Geometry check sheet. Reference: drawing and pictorial views, mm from the part's lowest x, y, z. Round coordinates to 2 decimals unless told otherwise and drop trailing zeros. Write each loop counter-clockwise with the first axis right and the second up, starting at its lowest first coordinate (ties: lowest second). Pieces come first, ordered by that corner, then holes. Notation, with made-up numbers: (-10.5, 33.5) -> (9.5, 33.5) arc R26 cw to (9.5, 47.5) -> close; hole circle Ø10 at (-8, 13). An arc over 180 degrees is marked (long way). Answer as a JSON object with one key per item and string values. Group by question number.
(1) Sectioned sample at D-D on x = 22. Record the cut outline in (y, z).
(2) Sectioned sample at A-A on x = 15.24. Record the cut outline in (y, z) (3 decimals).
(3) Draft check along X on the marked faces 1, 2, 3 and 4. Enter one of: released by +X, released by -X, zero draft, split by the parting line, or undercut.
(4) Scan lines: L1, parallel to Y at x = 15.24, z = 3.3 (3 decimals); L2, parallel to X at y = 28.5, z = 0.45; L3, parallel to X at y = 29.5, z = 3.4. Record each from-to range of solid material in increasing order. Write a range as from..to.
(5) Sectioned sample at B-B on z = 0.45. Record the cut outline in (x, y) (3 decimals), and give its area (3 significant figures).
(6) Gauge pin test, flat end, axial feed: pin 1 Ø1 at (x, z) = (18, 0.5) entering from -Y. Record the tip position at first contact, or that the pin passes through.
(7) Sectioned sample at C-C on y = 35.5. Record the cut outline in (x, z).
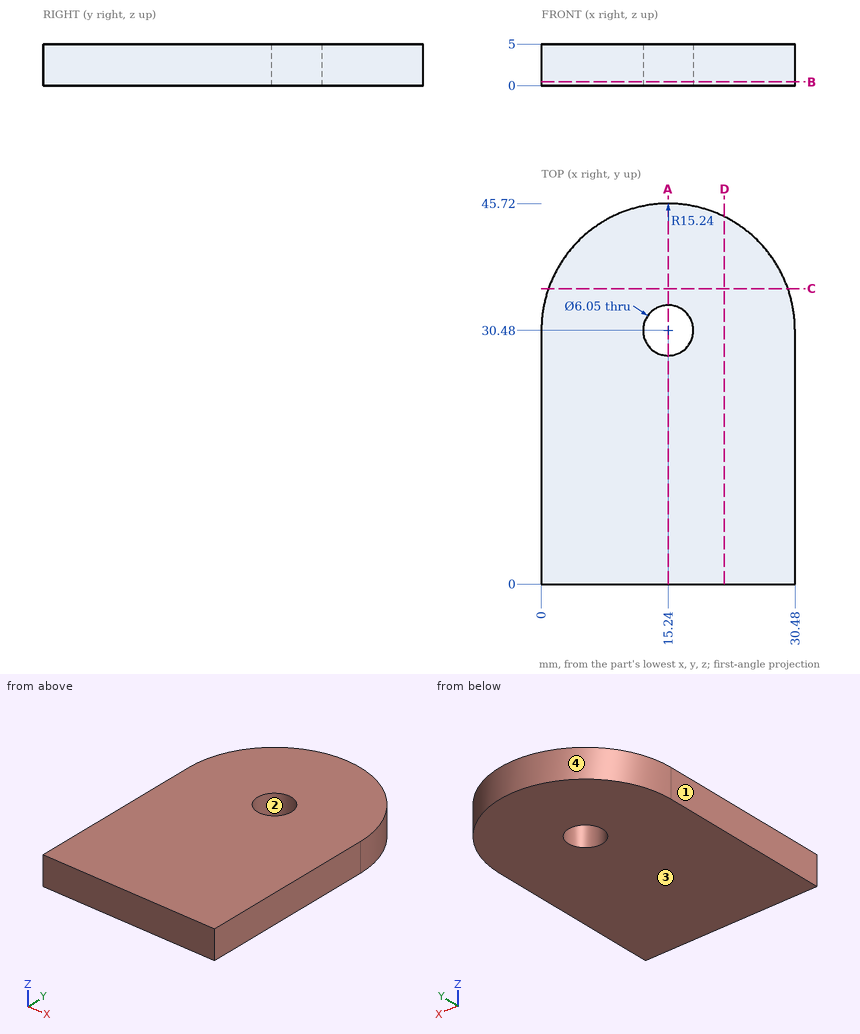
Computed values:
{
 "1": {"outline": "(0, 0) -> (44.14, 0) -> (44.14, 5) -> (0, 5) -> close"},
 "2": {"outline": "(0, 0) -> (27.455, 0) -> (27.455, 5) -> (0, 5) -> close; (33.505, 0) -> (45.72, 0) -> (45.72, 5) -> (33.505, 5) -> close"},
 "3": {"face 1": "released by -X", "face 2": "undercut", "face 3": "zero draft", "face 4": "split by the parting line"},
 "4": {"L1": "0..27.455, 33.505..45.72", "L2": "0..12.95, 17.53..30.48", "L3": "0..12.38, 18.1..30.48"},
 "5": {"outline": "(0, 0) -> (30.48, 0) -> (30.48, 30.48) arc R15.24 ccw to (0, 30.48) -> close; hole circle Ø6.05 at (15.24, 30.48)", "area": "1,270 mm2"},
 "6": {"pin 1": "y = 0"},
 "7": {"outline": "(0.85, 0) -> (29.63, 0) -> (29.63, 5) -> (0.85, 5) -> close"}
}
